Can you work these out from the model? Positions are in its coordinate system, mm. A direction names the side the tool comes from. Round coordinates to 2 decimals unless told otherwise and drop trailing zeros. Loops run counter-clockwise (first coordinate to the right, second up) from the corner with the lowest first, then second, coordinate; pieces in that order, holes last.
from build123d import *

# Parameters (mm, degrees)
SKETCH1_W           = 150
SKETCH1_H           = 150
SKETCH1_R           = 13.25
BOSS_EXTRUDE1_DEPTH = 15
SKETCH2_R           = 13.25
BOSS_EXTRUDE2_DEPTH = 8


with BuildPart() as part:
    # Sketch1 → Boss-Extrude1 (new body)
    with BuildSketch(Plane(origin=(0, 0, 0), x_dir=(1, 0, 0), z_dir=(0, 1, 0))):
        Rectangle(SKETCH1_W, SKETCH1_H)
        with Locations(Location((0, 0, 0), (0, 0, 270))):
            Circle(SKETCH1_R, mode=Mode.SUBTRACT)
    extrude(amount=BOSS_EXTRUDE1_DEPTH)

    # Sketch2 → Boss-Extrude2 (add)
    with BuildSketch(Plane.XZ):
        with Locations(Location((0, 0, 0), (0, 0, 270))):
            Circle(SKETCH2_R)
    extrude(amount=-BOSS_EXTRUDE2_DEPTH)


solid = part.part
(1) For faces 1 (the cylindrical face through (13.137, 11.451, -1.725)), 2 (the flat face through (-1, 7, -75)), which set-ups out of +Z, -Z, +X, -X, +Y, -Y let a thin tool reach every point of the face, with its end or its side?
Worked answers:
face 1: +Y
face 2: -Z, +X, -X, +Y, -Y
(2) If we section it at B-B, the plane x = 0: List the corners of the cut face in (y, z) for me, then the cut area to 3 significant figures.
Worked answers:
outline: (0, -75) - (15, -75) - (15, -13.25) - (8, -13.25) - (8, 13.25) - (15, 13.25) - (15, 75) - (0, 75) - close
area: 2,060 mm2
(3) If we section it at A-A, the plane z = 0: List the corners of the cut face in (x, y) for me, then the cut area to 3 significant figures.
Worked answers:
outline: (-75, 0) - (75, 0) - (75, 15) - (13.25, 15) - (13.25, 8) - (-13.25, 8) - (-13.25, 15) - (-75, 15) - close
area: 2,060 mm2
(4) If we mould it in two halves opening along X, with no side actions, what happens to faces 3 (the flat face through (0, 8, 0)), 4 (the flat face through (-75, 7, 1)), 5 (the flat face through (75, 7, 1)), 6 (the flat face through (-1, 15, -18))? For each: released by +X, released by -X, zero draft, split by the parting line, or undercut.
Worked answers:
face 3: undercut
face 4: released by -X
face 5: released by +X
face 6: zero draft
(5) Will these pins go through, and if not, where does the flat tip stop? P1, Ø21, axis at x = 0, z = 0, coming from the -Y side; P2, Ø13, axis at x = 2, z = -2, coming from the +Y side.
Worked answers:
P1: stops at y = 0
P2: stops at y = 8
(6) If I drill on line 1 (Z direction, x = 0, y = 10); line 2 (Z direction, x = -3, y = 10), over which ranges is the centre line in solid material (lowest first)?
Worked answers:
line 1: z = -75 to -13.25, 13.25 to 75
line 2: z = -75 to -12.91, 12.91 to 75
